```python
from build123d import *

# Parameters (mm, degrees)
PAD_DEPTH       = 40
SKETCH001_R     = 15
POCKET_DEPTH    = 74.001
FILLET_R        = 5
FILLET001_R     = 10
POCKET001_DEPTH = 5


with BuildPart() as part:
    # Sketch → Pad (new body)
    with BuildSketch(Plane.XY):
        Polygon((0, 0), (0, 123), (74, 123), (74, 0), (71, 0), (71, 120), (3, 120), (3, 0), align=None)
    extrude(amount=PAD_DEPTH)

    # Sketch001 → Pocket (cut, through all)
    with BuildSketch(Plane(origin=(0, 0, 0), x_dir=(0, -1, 0), z_dir=(-1, 0, 0))):
        with Locations((-23, 9.182545)):
            Circle(SKETCH001_R)
    extrude(amount=-POCKET_DEPTH, mode=Mode.SUBTRACT)

    # Fillet
    fillet_edges = [part.edges().sort_by_distance(p)[0] for p in [
        (0, 123, 20),
        (74, 123, 20),
        (71, 120, 20),
        (3, 120, 20),
    ]]
    fillet(fillet_edges, radius=FILLET_R)

    # Fillet001
    fillet001_edges = [part.edges().sort_by_distance(p)[0] for p in [
        (72.5, 0, 40),
        (1.5, 0, 40),
    ]]
    fillet(fillet001_edges, radius=FILLET001_R)

    # Sketch002 → Pocket001 (cut)
    with BuildSketch(Plane(origin=(0, 123, 0), x_dir=(-1, 0, 0), z_dir=(0, 1, 0))):
        with BuildLine():
            ThreePointArc((-38.291944, 15.429072), (-34.637435, 24.120775), (-40.291944, 16.575733))
            Line((-40.291944, 16.575733), (-40.291944, 0))
            Line((-40.291944, 0), (-38.291944, 0))
            Line((-38.291944, 0), (-38.291944, 15.429072))
        make_face()
    extrude(amount=-POCKET001_DEPTH, mode=Mode.SUBTRACT)


solid = part.part
```
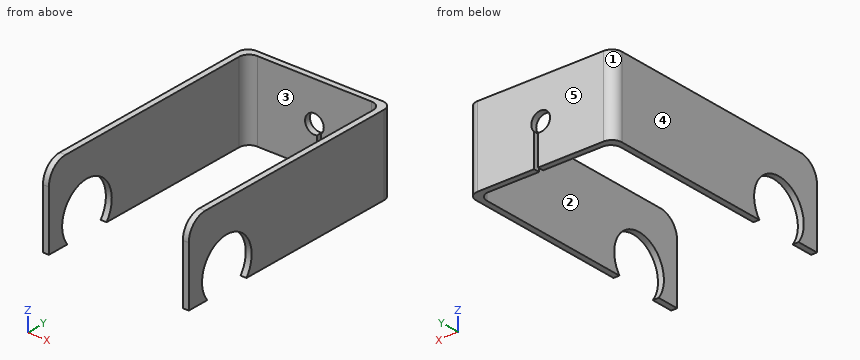
Verification items for the finished model (mm, model axes). Face numbers are marked on the shaded views. A direction names the side the tool comes from. Coordinates: 2 decimals unless noted, no trailing zeros. Write each loop counter-clockwise with the first axis right and the second up, starting at its lowest first coordinate (ties: lowest second). Pieces come first, ordered by that corner, then holes. Notation, with made-up numbers: M -31,75.5 L -21,75.5 A20 ccw -21,110.5 Z; hole C 14,-4.5 d9. An arc over 180 degrees is marked long. Answer as a JSON object with one key per item and string values. Group by question number.
(1) Tool access check on the marked faces 1 and 2. Record the directions out of +Z, -Z, +X, -X, +Y, -Y that give a thin tool (end or side, any length) a straight path to the whole face; none if there is none.
(2) Cross-section at B-B, the plane y = 46.5. Record the cut outline in (x, z), and give its area (3 significant figures).
(3) Cross-section at C-C, the plane z = 7. Record the cut outline in (x, y).
(4) Cross-section at D-D, the plane z = 20. Record the cut outline in (x, y).
(5) Material ranges on line 1 (X direction, y = 69, z = 18); line 2 (Y direction, x = 17.5, z = 35); line 3 (Z direction, x = 2.1, y = 23), recorded low to high.
(6) Cross-section at A-A, the plane x = 37. Record the cut outline in (y, z), and give its area (3 significant figures).
(7) Gauge pin test, flat ends, axial feed: pin 1 (2.5 mm diameter, centred on y = 121.5, z = 9, fed in from +X); pin 2 (20 mm diameter, centred on x = 30, z = 18, fed in from -Y); pin 3 (1.5 mm diameter, centred on y = 121.5, z = 4.5, fed in from -X). Record the tip position at first contact, or that the pin passes through.
(8) Release check for a two-part mould opening along X. For the marked faces 3, 4 and 5 record: +X half, -X half, draft (parallel to the pull), parting line (faces both ways), or undercut.
Reply:
{
 "1": {"face 1": "+Z, -Z, -X, +Y", "face 2": "+Z, -Z, -Y"},
 "2": {"outline": "M 0,0 L 3,0 L 3,40 L 0,40 Z; M 71,0 L 74,0 L 74,40 L 71,40 Z", "area": "240 mm²"},
 "3": {"outline": "M 0,0 L 3,0 L 3,8.16 L 0,8.16 Z; M 0,37.84 L 3,37.84 L 3,115 A5 cw 8,120 L 38.29,120 L 38.29,123 L 5,123 A5 ccw 0,118 Z; M 40.29,120 L 66,120 A5 cw 71,115 L 71,37.84 L 74,37.84 L 74,118 A5 ccw 69,123 L 40.29,123 Z; M 71,0 L 74,0 L 74,8.16 L 71,8.16 Z"},
 "4": {"outline": "M 0,0 L 3,0 L 3,12.61 L 0,12.61 Z; M 0,33.39 L 3,33.39 L 3,115 A5 cw 8,120 L 32.25,120 L 32.25,123 L 5,123 A5 ccw 0,118 Z; M 41.75,120 L 66,120 A5 cw 71,115 L 71,33.39 L 74,33.39 L 74,118 A5 ccw 69,123 L 41.75,123 Z; M 71,0 L 74,0 L 74,12.61 L 71,12.61 Z"},
 "5": {"line 1": "0 to 3, 71 to 74", "line 2": "120 to 123", "line 3": "24.18 to 40"},
 "6": {"outline": "M 120,0 L 123,0 L 123,15.25 L 120,15.25 Z; M 120,24.75 L 123,24.75 L 123,40 L 120,40 Z", "area": "91.5 mm²"},
 "7": {"pin 1": "x = 73.47", "pin 2": "y = 120", "pin 3": "x = 0.82"},
 "8": {"face 3": "undercut", "face 4": "-X half", "face 5": "draft"}
}
